For this review, take the finished solid that the model builds, in its own axes (mm). A direction names the side the tool comes from. Give positions to 0.01 mm unless a question says otherwise; leave off trailing zeros. Loops run counter-clockwise (first coordinate to the right, second up) from the corner with the lowest first, then second, coordinate; pieces in that order, holes last.
```python
from build123d import *

# Parameters (mm, degrees)
BOSS_EXTRUDE1_DEPTH = 5
BOSS_EXTRUDE2_DEPTH = 3
SKETCH3_R           = 10.5
CUT_EXTRUDE1_DEPTH  = 5
SKETCH4_R           = 2
CUT_EXTRUDE2_DEPTH  = 10
CIRPATTERN1_COUNT   = 3


with BuildPart() as part:
    # Sketch1 → Boss-Extrude1 (new body)
    with BuildSketch(Plane(origin=(0, 0, 0), x_dir=(1, 0, 0), z_dir=(0, 1, 0))):
        with BuildLine():
            Line((19, 0), (19, -15))
            Line((19, -15), (-19, -15))
            Line((-19, -15), (-19, 0))
            ThreePointArc((-19, 0), (0, 19), (19, 0))
        make_face()
    extrude(amount=BOSS_EXTRUDE1_DEPTH)

    # Sketch2 → Boss-Extrude2 (add)
    with BuildSketch(Plane.XY.offset(15)):
        with BuildLine():
            Line((-15, 4.482032097), (15, 4.482032097))
            ThreePointArc((15, 4.482032097), (17, 2.482032097), (15, 0.482032097))
            Line((15, 0.482032097), (-15, 0.482032097))
            ThreePointArc((-15, 0.482032097), (-17, 2.482032097), (-15, 4.482032097))
        make_face()
    extrude(amount=BOSS_EXTRUDE2_DEPTH)

    # Sketch3 → Cut-Extrude1 (cut)
    with BuildSketch(Plane(origin=(0, 5, 0), x_dir=(1, 0, 0), z_dir=(0, 1, 0))):
        with Locations(Location((0, 0, 0), (0, 0, 270))):
            Circle(SKETCH3_R)
    extrude(amount=-CUT_EXTRUDE1_DEPTH, mode=Mode.SUBTRACT)

    # Sketch4 → Cut-Extrude2 (cut)
    with BuildSketch(Plane(origin=(0, 5, 0), x_dir=(1, 0, 0), z_dir=(0, 1, 0))):
        with Locations(Location((0, 14, 0), (0, 0, 270))):
            Circle(SKETCH4_R)
    cut_extrude2 = extrude(amount=-CUT_EXTRUDE2_DEPTH, mode=Mode.SUBTRACT)

    # CirPattern1: Cut-Extrude2 ×3 about axis
    cirpattern1_axis = Axis((0, 0, 0), (0, 1, 0))
    for i in range(1, CIRPATTERN1_COUNT):
        add(cut_extrude2.rotate(cirpattern1_axis, i * 360 / CIRPATTERN1_COUNT), mode=Mode.SUBTRACT)


solid = part.part
```
Item 1: Take a section at B-B on z = -14. Give the boundary of the cut face in (x, y), and give its area (3 significant figures).
Answer:
outline: (-12.85, 0) - (-2, 0) - (-2, 5) - (-12.85, 5) - close; (2, 0) - (12.85, 0) - (12.85, 5) - (2, 5) - close
area: 108 mm2
Item 2: Take a section at D-D on z = 7. Give the boundary of the cut face in (x, y), and give its area (3 significant figures).
Answer:
outline: (-19, 0) - (-14.12, 0) - (-14.12, 5) - (-19, 5) - close; (-10.12, 0) - (-7.83, 0) - (-7.83, 5) - (-10.12, 5) - close; (7.83, 0) - (10.12, 0) - (10.12, 5) - (7.83, 5) - close; (14.12, 0) - (19, 0) - (19, 5) - (14.12, 5) - close
area: 71.7 mm2
Item 3: Clearance check with flat-ended pins moving along their axes: pin 1 Ø2.5 at (x, z) = (0, -14) entering from -Y; pin 2 Ø0.9 at (x, z) = (1.5, 16.5) entering from -Y; pin 3 Ø3 at (y, z) = (0.5, -13.5) entering from -X; pin 4 Ø1 at (x, y) = (0.5, 3) entering from -Z. State where each tip first meets the part, or that it passes through.
Answer:
pin 1: passes through
pin 2: stops at y = 0.48
pin 3: stops at x = -14.73
pin 4: stops at z = -19
Item 4: Tool access review of faces 5 (the cylindrical face through (-17, 2.4, 16.5)), 6 (the cylindrical face through (17, 2.5, 16.5)), 7 (the flat face through (9, 5, -6)), 8 (the flat face through (1.5, 0.3, 15)), 9 (the flat face through (0, 0.482, 16)): name each direction out of +Z, -Z, +X, -X, +Y, -Y from which nothing blocks a thin tool from reaching the whole face with its end or side.
Answer:
face 5: +Z, -X
face 6: +Z, +X
face 7: +Z, -Z, +X, -X, +Y
face 8: +Z
face 9: +Z, +X, -X, -Y
Item 5: Take a section at C-C on x = -9.5. Give the boundary of the cut face in (y, z).
Answer:
outline: (0, -16.45) - (5, -16.45) - (5, -4.47) - (0, -4.47) - close; (0, 4.47) - (5, 4.47) - (5, 15) - (4.48, 15) - (4.48, 18) - (0.48, 18) - (0.48, 15) - (0, 15) - close
Item 6: The part is to be moulded in two halves that separate along Z. For faces 1 (the cylindrical face through (0, 2, -19)), 2 (the cylindrical face through (3.2, 2.5, 10)), 3 (the flat face through (0, 4.482, 16)), 4 (the cylindrical face through (14.1, 2.5, 6.7)), say which applies: released by +Z, released by -Z, zero draft, split by the parting line, or undercut.
Answer:
face 1: released by -Z
face 2: undercut
face 3: zero draft
face 4: undercut
Item 7: Take a section at A-A on x = 0. Give the boundary of the cut face in (y, z), and give its area (3 significant figures).
Answer:
outline: (0, -19) - (5, -19) - (5, -16) - (0, -16) - close; (0, -12) - (5, -12) - (5, -10.5) - (0, -10.5) - close; (0, 10.5) - (5, 10.5) - (5, 15) - (4.48, 15) - (4.48, 18) - (0.48, 18) - (0.48, 15) - (0, 15) - close
area: 57.0 mm2
Item 8: For L1, parallel to X at y = 2.35, z = 7; L2, parallel to Y at x = -15, z = 16.5; L3, parallel to Z at x = 4.5, y = 2.5, list the stretches that pass through material, from the lowest coordinate up.
Answer:
L1: x = -19 to -14.12, -10.12 to -7.83, 7.83 to 10.12, 14.12 to 19
L2: y = 0.48 to 4.48
L3: z = -18.46 to -9.49, 9.49 to 18
